Read the model definition and answer for the solid it produces. Units are mm, in the model's axes. Give positions to 0.01 mm unless a question says otherwise; leave off trailing zeros. Write each loop counter-clockwise with the first axis right and the second up, starting at its lowest first coordinate (ties: lowest second). Pieces come first, ordered by that corner, then holes. Notation, with made-up numbers: (-12.5, 12.5) -> (2.5, 12.5) arc R14 ccw to (2.5, 21.5) -> close; hole circle Ø10 at (-8, 26). An arc over 180 degrees is marked (long way). Use a Markdown table: item, result.
Autodesk Inventor part; units mm, degrees
ref_plane "YZ Plane" through (0, 0, 0) normal (1, 0, 0) x (0, 1, 0)
ref_plane "XZ Plane" through (0, 0, 0) normal (0, 1, 0) x (-1, 0, 0)
ref_plane "XY Plane" through (0, 0, 0) normal (0, 0, 1) x (1, 0, 0)
sketch "Sketch2" plane through (0, 0, 0) normal (0, 1, 0) x (-1, 0, 0)
  circle A0 centre (0, 0) radius 16.75
  circle A1 centre (0, 0) radius 25
  circle A2 centre (0, 0) radius 31
  circle A3 centre (25, 0) radius 3
  circle A4 centre (0, 25) radius 3
  circle A5 centre (0, -25) radius 3
  circle A6 centre (-25, 0) radius 3
  circle A7 centre (17.6777, -17.6777) radius 3
  line L0 (0, 0) -> (25, 0)
  line L1 (0, 0) -> (17.6777, -17.6777)
  dimension "d0" = 33.5
  dimension "d1" = 50
  dimension "d2" = 62
  dimension "d3" = 6
  dimension "d4" = 6
  dimension "d5" = 45
extrude "Extrusion1" add sketch "Sketch2" along normal blind 3 contours L0 A3 A1 A7 L1 A0 | A0 L1 A7 A1 A5 A6 A4 A3 L0 | A2
properties part number "robotiq_ur5_flange_adapter_flattener"
Item 1: A cutting plane is placed at D-D (z = 25). Give the vertices of the cut face in (x, y).
Return value:
| item | result |
|---|---|
| outline | (-18.33, 0) -> (-3, 0) -> (-3, 3) -> (-18.33, 3) -> close; (3, 0) -> (18.33, 0) -> (18.33, 3) -> (3, 3) -> close |
Item 2: A cutting plane is placed at C-C (x = -25). Give the vertices of the cut face in (y, z), then the cut area to 3 significant figures.
Return value:
| item | result |
|---|---|
| outline | (0, -18.33) -> (3, -18.33) -> (3, -3) -> (0, -3) -> close; (0, 3) -> (3, 3) -> (3, 18.33) -> (0, 18.33) -> close |
| area | 92.0 mm^2 |
Item 3: A cutting plane is placed at B-B (z = 0). Give the vertices of the cut face in (x, y), then the cut area to 3 significant figures.
Return value:
| item | result |
|---|---|
| outline | (-31, 0) -> (-28, 0) -> (-28, 3) -> (-31, 3) -> close; (-22, 0) -> (-16.75, 0) -> (-16.75, 3) -> (-22, 3) -> close; (16.75, 0) -> (22, 0) -> (22, 3) -> (16.75, 3) -> close; (28, 0) -> (31, 0) -> (31, 3) -> (28, 3) -> close |
| area | 49.5 mm^2 |
Item 4: Each of these flat-tipped pins is pushed along its axis until it touches: P1, Ø5.5, axis at x = 0, z = -25, coming from the +Y side; P2, Ø1.5, axis at y = 1.5, z = 5.5, coming from the +X side; P3, Ø1.5, axis at x = -3.5, y = 1.5, coming from the -Z side. Where does it stop, or does it pass through?
Return value:
| item | result |
|---|---|
| P1 | through |
| P2 | x = 30.63 |
| P3 | z = -30.88 |
Item 5: A cutting plane is placed at A-A (x = 0). Give the vertices of the cut face in (y, z), then the cut area to 3 significant figures.
Return value:
| item | result |
|---|---|
| outline | (0, -31) -> (3, -31) -> (3, -28) -> (0, -28) -> close; (0, -22) -> (3, -22) -> (3, -16.75) -> (0, -16.75) -> close; (0, 16.75) -> (3, 16.75) -> (3, 22) -> (0, 22) -> close; (0, 28) -> (3, 28) -> (3, 31) -> (0, 31) -> close |
| area | 49.5 mm^2 |
Item 6: For a pull along Z with two mould halves and no side action, classify faces 1 (the face through (-13, 3, -13)), 2 (the face through (4.036, 1.479, -30.736)), 3 (the face through (3.63, 1.48, 16.35)) as +Z half, -Z half, draft (parallel to the pull), parting line (faces both ways), or undercut.
Return value:
| item | result |
|---|---|
| face 1 | draft |
| face 2 | parting line |
| face 3 | undercut |
Item 7: Straight lines are drawn through the part: line 1 along Z through (x, y) = (0, 1.85); line 2 along Z through (x, y) = (-15, 2.05); line 3 along X through (y, z) = (0.7, -25). For each, find the intervals that lie inside material, in ascending order. Write a range as [from, to].
Return value:
| item | result |
|---|---|
| line 1 | [-31, -28], [-22, -16.75], [16.75, 22], [28, 31] |
| line 2 | [-27.13, -19.03], [-16.32, -7.45], [7.45, 27.13] |
| line 3 | [-18.33, -3], [3, 18.33] |
